Part model, mm, in its own coordinate system. Face numbers are marked on the shaded views. A direction names the side the tool comes from. Coordinates: 2 decimals unless noted, no trailing zeros. Loops run counter-clockwise (first coordinate to the right, second up) from the corner with the lowest first, then second, coordinate; pieces in that order, holes last. Notation, with made-up numbers: (59.25, -6) - (108.25, -6) arc R19 ccw to (108.25, 14) - close; hole circle Ø1 at (-26, 45). An arc over 180 degrees is marked (long way). Answer as CSV lines item,"result".
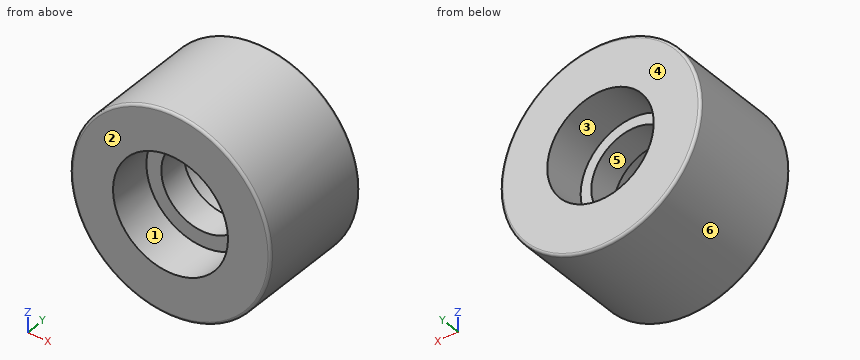
from build123d import *


with BuildPart() as part:
    # Szkic1 → Obrót1 (revolve)
    with BuildSketch(Plane.XY, mode=Mode.PRIVATE) as obr_t1_sk:
        with BuildLine():
            Line((-12.5, 28), (-22.9, 28))
            ThreePointArc((-22.9, 28), (-23.324264069, 27.824264069), (-23.5, 27.4))
            Line((-23.5, 27.4), (-23.5, 0.6))
            ThreePointArc((-23.5, 0.6), (-23.324264069, 0.175735931), (-22.9, 0))
            Line((-22.9, 0), (-13.5, 0))
            Line((-13.5, 0), (-13.5, 10.5))
            Line((-13.5, 10.5), (-10, 10.5))
            Line((-10, 10.5), (-10, 17.5))
            Line((-10, 17.5), (-12.5, 17.5))
            Line((-12.5, 17.5), (-12.5, 28))
        make_face()
    revolve(obr_t1_sk.sketch.rotate(Axis((0, 0, 0), (0, 1, 0)), 180), axis=Axis((0, 0, 0), (0, 1, 0)))


solid = part.part
Q1. Wall check: L1, parallel to Z at x = 0, y = 8.75; L2, parallel to Z at x = 0, y = 25.75; L3, parallel to X at y = 8.25, z = 7. Give the ranges that are in metal, low to high.
Results:
L1,"z = -23.5 to -13.5, 13.5 to 23.5"
L2,"z = -23.5 to -12.5, 12.5 to 23.5"
L3,"x = -22.43 to -11.54, 11.54 to 22.43"
Q2. Saw through at D-D (y = 3). Give the cut face in (x, z), then the cut area to 3 significant figures.
Results:
outline,"circle Ø47 at (0, 0); hole circle Ø27 at (0, 0)"
area,"1,160 mm^2"
Q3. Saw through at C-C (y = 23.25). Give the cut face in (x, z).
Results:
outline,"circle Ø47 at (0, 0); hole circle Ø25 at (0, 0)"
Q4. Which spindle directions (+Z, -Z, +X, -X, +Y, -Y) get a long thin tool onto all of the face, cutting with end or side? Do the marked faces 1, 2 and 3. Say none if no direction does.
Results:
face 1,"-Y"
face 2,"+Z, -Z, +X, -X, -Y"
face 3,"+Y"
Q5. Two-plate mould, pull along Z, no slides. Class the marked faces 4, 5 and 6: released by +Z, released by -Z, zero draft, split by the parting line, or undercut.
Results:
face 4,"zero draft"
face 5,"undercut"
face 6,"split by the parting line"
Q6. Saw through at B-B (z = 0). Give the cut face in (x, y), then the cut area to 3 significant figures.
Results:
outline,"(-23.5, 0.6) arc R0.6 ccw to (-22.9, 0) - (-13.5, 0) - (-13.5, 10.5) - (-10, 10.5) - (-10, 17.5) - (-12.5, 17.5) - (-12.5, 28) - (-22.9, 28) arc R0.6 ccw to (-23.5, 27.4) - close; (10, 10.5) - (13.5, 10.5) - (13.5, 0) - (22.9, 0) arc R0.6 ccw to (23.5, 0.6) - (23.5, 27.4) arc R0.6 ccw to (22.9, 28) - (12.5, 28) - (12.5, 17.5) - (10, 17.5) - close"
area,"630 mm^2"
Q7. Saw through at A-A (x = 0). Give the cut face in (y, z), then the cut area to 3 significant figures.
Results:
outline,"(0, -22.9) arc R0.6 ccw to (0.6, -23.5) - (27.4, -23.5) arc R0.6 ccw to (28, -22.9) - (28, -12.5) - (17.5, -12.5) - (17.5, -10) - (10.5, -10) - (10.5, -13.5) - (0, -13.5) - close; (0, 13.5) - (10.5, 13.5) - (10.5, 10) - (17.5, 10) - (17.5, 12.5) - (28, 12.5) - (28, 22.9) arc R0.6 ccw to (27.4, 23.5) - (0.6, 23.5) arc R0.6 ccw to (0, 22.9) - close"
area,"630 mm^2"
Q8. Flat gauge pins, fed straight in: pin 1 (12 mm diameter, centred on x = -10, y = 3.5, fed in from -Z); pin 2 (1 mm diameter, centred on y = 24, z = -14, fed in from +X); pin 3 (1 mm diameter, centred on x = 4, y = 16, fed in from +Z). Where does each tip first touch, or does it go through?
Results:
pin 1,"stops at z = -23.16"
pin 2,"stops at x = 19.24"
pin 3,"stops at z = 23.24"
